```python
from build123d import *

# Parameters (mm, degrees)
SKETCH1_R                   = 1.15
SHAPE_DEPTH                 = 0.5
CAMERA_CONNECTOR_HOLE_REACH = 32.927
FILLET1_R                   = 2


with BuildPart() as part:
    # Sketch1 → Shape (new body)
    # profile 1 of 2: a face of its own
    with BuildSketch(Plane.XY):
        with BuildLine():
            Line((17.5, -7.325), (19.5, -7.325))
            Line((19.5, -7.325), (19.5, 4.675))
            Line((19.5, 4.675), (17.5, 4.675))
            Line((17.5, 4.675), (17.5, 9.4))
            ThreePointArc((17.5, 9.4), (17.280330086, 9.930330086), (16.75, 10.15))
            Line((16.75, 10.15), (13.05, 10.15))
            ThreePointArc((13.05, 10.15), (12.519669914, 10.369669914), (12.3, 10.9))
            Line((12.3, 10.9), (12.3, 14.15))
            ThreePointArc((12.3, 14.15), (12.080330086, 14.680330086), (11.55, 14.9))
            Line((11.55, 14.9), (9.2, 14.9))
            ThreePointArc((9.2, 14.9), (7.760617121, 15.452916118), (7.061567259, 16.827277277))
            ThreePointArc((7.061567259, 16.827277277), (6.817712656, 17.306705589), (6.315602349, 17.499583304))
            Line((6.315602349, 17.499583304), (-11.55, 17.499583304))
            ThreePointArc((-11.55, 17.499583304), (-12.080330086, 17.27991339), (-12.3, 16.749583304))
            Line((-12.3, 16.749583304), (-12.3, 10.9))
            ThreePointArc((-12.3, 10.9), (-12.519669914, 10.369669914), (-13.05, 10.15))
            Line((-13.05, 10.15), (-16.75, 10.15))
            ThreePointArc((-16.75, 10.15), (-17.280330086, 9.930330086), (-17.5, 9.4))
            Line((-17.5, 9.4), (-17.5, -9.4))
            ThreePointArc((-17.5, -9.4), (-17.280330086, -9.930330086), (-16.75, -10.15))
            Line((-16.75, -10.15), (-13.05, -10.15))
            ThreePointArc((-13.05, -10.15), (-12.519669914, -10.369669914), (-12.3, -10.9))
            Line((-12.3, -10.9), (-12.3, -16.749583304))
            ThreePointArc((-12.3, -16.749583304), (-12.080330086, -17.27991339), (-11.55, -17.499583304))
            Line((-11.55, -17.499583304), (11.55, -17.499583304))
            ThreePointArc((11.55, -17.499583304), (12.080330086, -17.27991339), (12.3, -16.749583304))
            Line((12.3, -16.749583304), (12.3, -10.9))
            ThreePointArc((12.3, -10.9), (12.519669914, -10.369669914), (13.05, -10.15))
            Line((13.05, -10.15), (16.75, -10.15))
            ThreePointArc((16.75, -10.15), (17.280330086, -9.930330086), (17.5, -9.4))
            Line((17.5, -9.4), (17.5, -7.325))
        make_face()
    # profile 2 of 2: a face of its own
    with BuildSketch(Plane.XY):
        with BuildLine():
            Line((19.5, -19.5), (19.5, -7.325))
            Line((19.5, -7.325), (17.5, -7.325))
            Line((17.5, -7.325), (17.5, -9.4))
            ThreePointArc((17.5, -9.4), (17.280330086, -9.930330086), (16.75, -10.15))
            Line((16.75, -10.15), (13.05, -10.15))
            ThreePointArc((13.05, -10.15), (12.519669914, -10.369669914), (12.3, -10.9))
            Line((12.3, -10.9), (12.3, -16.749583304))
            ThreePointArc((12.3, -16.749583304), (12.080330086, -17.27991339), (11.55, -17.499583304))
            Line((11.55, -17.499583304), (-11.55, -17.499583304))
            ThreePointArc((-11.55, -17.499583304), (-12.080330086, -17.27991339), (-12.3, -16.749583304))
            Line((-12.3, -16.749583304), (-12.3, -10.9))
            ThreePointArc((-12.3, -10.9), (-12.519669914, -10.369669914), (-13.05, -10.15))
            Line((-13.05, -10.15), (-16.75, -10.15))
            ThreePointArc((-16.75, -10.15), (-17.280330086, -9.930330086), (-17.5, -9.4))
            Line((-17.5, -9.4), (-17.5, 9.4))
            ThreePointArc((-17.5, 9.4), (-17.280330086, 9.930330086), (-16.75, 10.15))
            Line((-16.75, 10.15), (-13.05, 10.15))
            ThreePointArc((-13.05, 10.15), (-12.519669914, 10.369669914), (-12.3, 10.9))
            Line((-12.3, 10.9), (-12.3, 16.749583304))
            ThreePointArc((-12.3, 16.749583304), (-12.080330086, 17.27991339), (-11.55, 17.499583304))
            Line((-11.55, 17.499583304), (6.315602349, 17.499583304))
            ThreePointArc((6.315602349, 17.499583304), (6.817712656, 17.306705589), (7.061567259, 16.827277277))
            ThreePointArc((7.061567259, 16.827277277), (7.760617121, 15.452916118), (9.2, 14.9))
            Line((9.2, 14.9), (11.55, 14.9))
            ThreePointArc((11.55, 14.9), (12.080330086, 14.680330086), (12.3, 14.15))
            Line((12.3, 14.15), (12.3, 10.9))
            ThreePointArc((12.3, 10.9), (12.519669914, 10.369669914), (13.05, 10.15))
            Line((13.05, 10.15), (16.75, 10.15))
            ThreePointArc((16.75, 10.15), (17.280330086, 9.930330086), (17.5, 9.4))
            Line((17.5, 9.4), (17.5, 4.675))
            Line((17.5, 4.675), (19.5, 4.675))
            Line((19.5, 4.675), (19.5, 24))
            Line((19.5, 24), (-19.5, 24))
            Line((-19.5, 24), (-19.5, -19.5))
            Line((-19.5, -19.5), (-16.775, -19.5))
            Line((-16.775, -19.5), (-16.775, -15.734122918))
            ThreePointArc((-16.775, -15.734122918), (-16.85, -15.25), (-16.775, -14.765877082))
            Line((-16.775, -14.765877082), (-16.775, -12.610660172))
            ThreePointArc((-16.775, -12.610660172), (-16.937579563, -11.793317512), (-16.244669914, -11.330330086))
            Line((-16.244669914, -11.330330086), (-15.505330086, -11.330330086))
            ThreePointArc((-15.505330086, -11.330330086), (-14.812420437, -11.793317512), (-14.975, -12.610660172))
            Line((-14.975, -12.610660172), (-14.975, -13.673809973))
            ThreePointArc((-14.975, -13.673809973), (-13.65, -15.25), (-14.975, -16.826190027))
            Line((-14.975, -16.826190027), (-14.975, -19.5))
            Line((-14.975, -19.5), (14.975, -19.5))
            Line((14.975, -19.5), (14.975, -16.826190027))
            ThreePointArc((14.975, -16.826190027), (13.65, -15.25), (14.975, -13.673809973))
            Line((14.975, -13.673809973), (14.975, -12.610660172))
            ThreePointArc((14.975, -12.610660172), (14.812420437, -11.793317512), (15.505330086, -11.330330086))
            Line((15.505330086, -11.330330086), (16.244669914, -11.330330086))
            ThreePointArc((16.244669914, -11.330330086), (16.937579563, -11.793317512), (16.775, -12.610660172))
            Line((16.775, -12.610660172), (16.775, -14.765877082))
            ThreePointArc((16.775, -14.765877082), (16.85, -15.25), (16.775, -15.734122918))
            Line((16.775, -15.734122918), (16.775, -19.5))
            Line((16.775, -19.5), (19.5, -19.5))
        make_face()
        with BuildLine():
            Line((-16.775, 12.610660172), (-16.775, 14.765877082))
            ThreePointArc((-16.775, 14.765877082), (-16.85, 15.25), (-16.775, 15.734122918))
            Line((-16.775, 15.734122918), (-16.775, 21.539339828))
            ThreePointArc((-16.775, 21.539339828), (-16.937579563, 22.356682488), (-16.244669914, 22.819669914))
            Line((-16.244669914, 22.819669914), (-15.505330086, 22.819669914))
            ThreePointArc((-15.505330086, 22.819669914), (-14.812420437, 22.356682488), (-14.975, 21.539339828))
            Line((-14.975, 21.539339828), (-14.975, 16.826190027))
            ThreePointArc((-14.975, 16.826190027), (-13.65, 15.25), (-14.975, 13.673809973))
            Line((-14.975, 13.673809973), (-14.975, 12.610660172))
            ThreePointArc((-14.975, 12.610660172), (-14.812420437, 11.793317512), (-15.505330086, 11.330330086))
            Line((-15.505330086, 11.330330086), (-16.244669914, 11.330330086))
            ThreePointArc((-16.244669914, 11.330330086), (-16.937579563, 11.793317512), (-16.775, 12.610660172))
        make_face(mode=Mode.SUBTRACT)
        with Locations((9.2, 17.05)):
            Circle(SKETCH1_R, mode=Mode.SUBTRACT)
        with BuildLine():
            Line((14.975, 12.610660172), (14.975, 13.673809973))
            ThreePointArc((14.975, 13.673809973), (13.65, 15.25), (14.975, 16.826190027))
            Line((14.975, 16.826190027), (14.975, 21.539339828))
            ThreePointArc((14.975, 21.539339828), (14.812420437, 22.356682488), (15.505330086, 22.819669914))
            Line((15.505330086, 22.819669914), (16.244669914, 22.819669914))
            ThreePointArc((16.244669914, 22.819669914), (16.937579563, 22.356682488), (16.775, 21.539339828))
            Line((16.775, 21.539339828), (16.775, 15.734122918))
            ThreePointArc((16.775, 15.734122918), (16.85, 15.25), (16.775, 14.765877082))
            Line((16.775, 14.765877082), (16.775, 12.610660172))
            ThreePointArc((16.775, 12.610660172), (16.937579563, 11.793317512), (16.244669914, 11.330330086))
            Line((16.244669914, 11.330330086), (15.505330086, 11.330330086))
            ThreePointArc((15.505330086, 11.330330086), (14.812420437, 11.793317512), (14.975, 12.610660172))
        make_face(mode=Mode.SUBTRACT)
    extrude(amount=SHAPE_DEPTH)

    # Sketch2 → Camera connector hole (cut, up to next)
    with BuildSketch(Plane.XY.offset(0.5), mode=Mode.PRIVATE) as camera_connector_hole_sk1:
        with BuildLine():
            Line((2.05, -0.698177871), (7.55, -0.698177871))
            ThreePointArc((7.55, -0.698177871), (8.080330086, -0.478507957), (8.3, 0.051822129))
            Line((8.3, 0.051822129), (8.3, 2.051822129))
            ThreePointArc((8.3, 2.051822129), (8.080330086, 2.582152215), (7.55, 2.801822129))
            Line((7.55, 2.801822129), (2.05, 2.801822129))
            ThreePointArc((2.05, 2.801822129), (1.519669914, 2.582152215), (1.3, 2.051822129))
            Line((1.3, 2.051822129), (1.3, 0.051822129))
            ThreePointArc((1.3, 0.051822129), (1.519669914, -0.478507957), (2.05, -0.698177871))
        make_face()
    camera_connector_hole_tool1 = extrude(camera_connector_hole_sk1.sketch, amount=-CAMERA_CONNECTOR_HOLE_REACH, mode=Mode.PRIVATE) & part.part
    add(camera_connector_hole_tool1.solids().sort_by_distance((4.8, 1.051822, 0.5))[0], mode=Mode.SUBTRACT)

    # Fillet1
    fillet1_edges = [part.edges().sort_by_distance(p)[0] for p in [
        (-19.5, 24, 0.25),
        (19.5, 24, 0.25),
    ]]
    fillet(fillet1_edges, radius=FILLET1_R)


solid = part.part
```
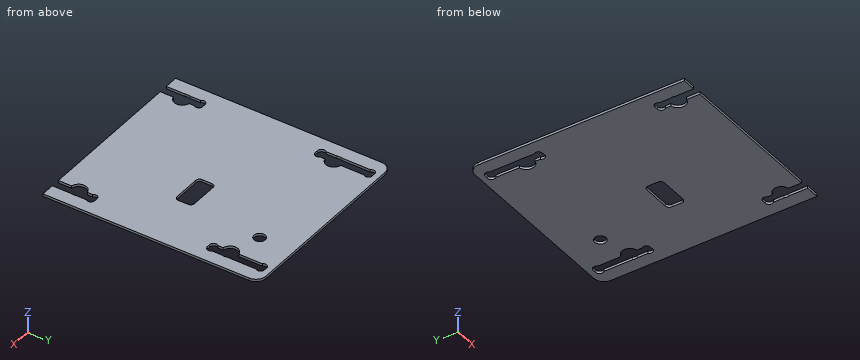
Read the model definition and answer for the solid it produces. Units are mm, in the model's axes. Coordinates: 2 decimals unless noted, no trailing zeros. Order: outer loops, then holes, each group sorted by start corner. A loop starts at its lowest first (then second) coordinate and runs counter-clockwise, first axis right, second up. Notation, with made-up numbers: (15.5, 28) - (55.5, 28) arc R20 cw to (55.5, 36) - close; hole circle Ø6 at (0.25, -29). An arc over 180 degrees is marked (long way). Answer as a JSON object with one key per item and string values. Group by question number.
Item 1: Section B-B (z = 0.15) is taken. State how many separate pieces and enclosed holes the cut face has, plus the area to 3 significant figures.
Item 2: Consider probe 1 along Y at (x, z) = (9.2, 0.2); probe 2 along X at (y, z) = (-15, 0.3); probe 3 along X at (y, z) = (18, 0.35) (3 decimals). Determine where each line is inside the solid, lowest interval first. Write a range as from..to.
Item 3: Section A-A (x = 9.2) is taken. Give the vertices of the cut face in (y, z).
Results are:
{
 "1": {"separate pieces": "1", "enclosed holes": "4", "area": "1,580 mm^2"},
 "2": {"probe 1": "y = -19.5..15.9, 18.2..24", "probe 2": "x = -19.5..-16.83, -13.67..13.67, 16.83..19.5", "probe 3": "x = -19.5..-16.775, -14.975..8.552, 9.848..14.975, 16.775..19.5"},
 "3": {"outline": "(-19.5, 0) - (15.9, 0) - (15.9, 0.5) - (-19.5, 0.5) - close; (18.2, 0) - (24, 0) - (24, 0.5) - (18.2, 0.5) - close"}
}
